```python
from build123d import *

# Parameters (mm, degrees)
SKETCH1_W           = 8
SKETCH1_H           = 8
BOSS_EXTRUDE1_DEPTH = 9.6
SKETCH2_R           = 2.4
BOSS_EXTRUDE2_DEPTH = 1.6
SHELL1_T            = -1.6


with BuildPart() as part:
    # Sketch1 → Boss-Extrude1 (new body)
    with BuildSketch(Plane(origin=(0, 0, 0), x_dir=(1, 0, 0), z_dir=(0, 1, 0))):
        with Locations((4, 4)):
            Rectangle(SKETCH1_W, SKETCH1_H)
    extrude(amount=BOSS_EXTRUDE1_DEPTH)

    # Sketch2 → Boss-Extrude2 (add)
    with BuildSketch(Plane(origin=(0, 9.6, 0), x_dir=(1, 0, 0), z_dir=(0, 1, 0))):
        with Locations(Location((4, 4, 0), (0, 0, 270))):
            Circle(SKETCH2_R)
    extrude(amount=BOSS_EXTRUDE2_DEPTH)

    # Shell1
    shell1_openings = [part.faces().sort_by_distance(p)[0] for p in [
        (4, 0, -4),
    ]]
    offset(amount=SHELL1_T, openings=shell1_openings, kind=Kind.INTERSECTION)


solid = part.part
```
Here's how the part is built. I have some questions about the finished solid (model axes, mm). A direction names the side the tool comes from. Coordinates: 2 decimals unless noted, no trailing zeros. Loops run counter-clockwise (first coordinate to the right, second up) from the corner with the lowest first, then second, coordinate; pieces in that order, holes last. Notation, with made-up numbers: (-40, 57) -> (-16, 57) arc R15 cw to (-16, 61) -> close; hole circle Ø8 at (-17, -26.75). An arc over 180 degrees is marked (long way). Return JSON: item names as keys, results as strings.
1) Thinking about a two-plate mould opening in Z: for faces 1 (the face through (4, 9.6, -4)), 2 (the face through (6.024, 10.389, -2.71)), 3 (the face through (4, 5, 0)), which applies, +Z half, -Z half, draft (parallel to the pull), parting line (faces both ways), or undercut?
Results below:
{"face 1": "undercut", "face 2": "parting line", "face 3": "+Z half"}
2) If we section it at A-A, the plane z = -4: Write out the boundary of the cut face in (x, y).
Results below:
{"outline": "(0, 0) -> (1.6, 0) -> (1.6, 8) -> (3.2, 8) -> (3.2, 9.6) -> (4.8, 9.6) -> (4.8, 8) -> (6.4, 8) -> (6.4, 0) -> (8, 0) -> (8, 9.6) -> (6.4, 9.6) -> (6.4, 11.2) -> (1.6, 11.2) -> (1.6, 9.6) -> (0, 9.6) -> close"}
3) For faces 4 (the face through (6, 9.6, -2)), 5 (the face through (1.6, 4, -4)), 6 (the face through (4, 11.2, -4)), which set-ups out of +Z, -Z, +X, -X, +Y, -Y let a thin tool reach every point of the face, with its end or its side?
Results below:
{"face 4": "+Y", "face 5": "-Y", "face 6": "+Z, -Z, +X, -X, +Y"}
4) If we section it at C-C, the plane x = 4: Write out the boundary of the cut face in (y, z), then the cut area to 3 significant figures.
Results below:
{"outline": "(0, -8) -> (9.6, -8) -> (9.6, -6.4) -> (11.2, -6.4) -> (11.2, -1.6) -> (9.6, -1.6) -> (9.6, 0) -> (0, 0) -> (0, -1.6) -> (8, -1.6) -> (8, -3.2) -> (9.6, -3.2) -> (9.6, -4.8) -> (8, -4.8) -> (8, -6.4) -> (0, -6.4) -> close", "area": "43.5 mm²"}
5) If we section it at D-D, the plane y = 9: Write out the boundary of the cut face in (x, z), then the cut area to 3 significant figures.
Results below:
{"outline": "(0, -8) -> (8, -8) -> (8, 0) -> (0, 0) -> close; hole circle Ø1.6 at (4, -4)", "area": "62.0 mm²"}
6) I need wall thicknesses on line 1 (Z direction, x = 4, y = 8.7); line 2 (X direction, y = 4.5, z = -2.75); line 3 (Z direction, x = 3.75, y = 6.5). Which ranges of each line are inside material? Lowest first, please. Write a range as from..to.
Results below:
{"line 1": "-8..-4.8, -3.2..0", "line 2": "0..1.6, 6.4..8", "line 3": "-8..-6.4, -1.6..0"}
7) If we section it at B-B, the plane y = 4.25: Write out the boundary of the cut face in (x, z).
Results below:
{"outline": "(0, -8) -> (8, -8) -> (8, 0) -> (0, 0) -> close; hole (1.6, -6.4) -> (6.4, -6.4) -> (6.4, -1.6) -> (1.6, -1.6) -> close"}
8) Will these pins go through, and if not, where does the flat tip stop? pin 1 (0.8 mm diameter, centred on x = 4, z = -3.5, fed in from -Y); pin 2 (1.3 mm diameter, centred on x = 4, z = -4, fed in from -Y).
Results below:
{"pin 1": "y = 8", "pin 2": "y = 9.6"}
